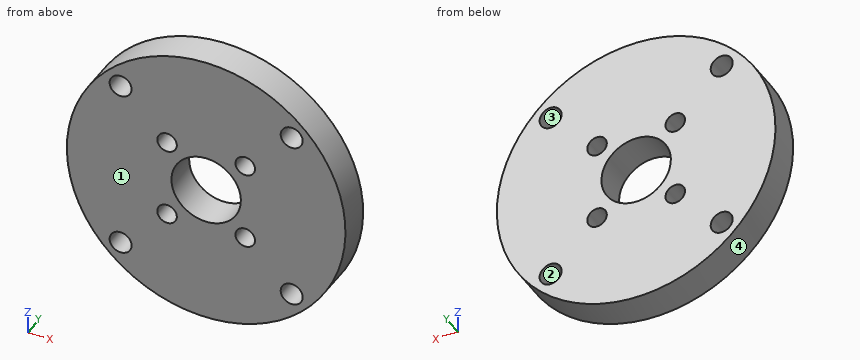
```python
from build123d import *

# Parameters (mm, degrees)
SKETCH1_R           = 28.5
BOSS_EXTRUDE1_DEPTH = 3.5
SKETCH2_R           = 2.25
SKETCH2_R_2         = 2
CUT_EXTRUDE1_DEPTH  = 41.908434338
SKETCH3_R           = 7.1
CUT_EXTRUDE2_DEPTH  = 41.908434338


with BuildPart() as part:
    # Sketch1 → Boss-Extrude1 (new, symmetric)
    with BuildSketch(Plane(origin=(0, 0, 0), x_dir=(1, 0, 0), z_dir=(0, 1, 0))):
        with Locations(Location((0, 0, 0), (0, 0, 270))):
            Circle(SKETCH1_R)
    extrude(amount=BOSS_EXTRUDE1_DEPTH, both=True)

    # Sketch2 → Cut-Extrude1 (cut, through all)
    with BuildSketch(Plane(origin=(0, 3.5, 0), x_dir=(1, 0, 0), z_dir=(0, 1, 0))):
        with Locations(Location((17.500892834, 17.500892834, 0), (0, 0, 270))):
            Circle(SKETCH2_R)
        with Locations(Location((17.500892834, -17.500892834, 0), (0, 0, 270))):
            Circle(SKETCH2_R)
        with Locations(Location((-17.500892834, -17.500892834, 0), (0, 0, 270))):
            Circle(SKETCH2_R)
        with Locations(Location((-17.500892834, 17.500892834, 0), (0, 0, 270))):
            Circle(SKETCH2_R)
        with Locations(Location((-8, -8, 0), (0, 0, 270))):
            Circle(SKETCH2_R_2)
        with Locations(Location((-8, 8, 0), (0, 0, 270))):
            Circle(SKETCH2_R_2)
        with Locations(Location((8, 8, 0), (0, 0, 270))):
            Circle(SKETCH2_R_2)
        with Locations(Location((8, -8, 0), (0, 0, 270))):
            Circle(SKETCH2_R_2)
    extrude(amount=-CUT_EXTRUDE1_DEPTH, mode=Mode.SUBTRACT)

    # Sketch3 → Cut-Extrude2 (cut, through all)
    with BuildSketch(Plane(origin=(0, 3.5, 0), x_dir=(1, 0, 0), z_dir=(0, 1, 0))):
        with Locations(Location((0, 0, 0), (0, 0, 270))):
            Circle(SKETCH3_R)
    extrude(amount=-CUT_EXTRUDE2_DEPTH, mode=Mode.SUBTRACT)


solid = part.part
```
Design review of the part built by this model. Coordinates are the model's own, in mm. Face numbers are marked on the shaded views. Coordinates: 2 decimals unless noted, no trailing zeros. Loops run counter-clockwise (first coordinate to the right, second up) from the corner with the lowest first, then second, coordinate; pieces in that order, holes last. Notation, with made-up numbers: (28.5, 47) - (45.5, 47) arc R23 cw to (45.5, 60) - close; hole circle Ø4 at (-6, 31). An arc over 180 degrees is marked (long way). Use CSV: the item, a comma, the result in double quotes. Start each with the question number.
1) Consider section A-A on x = 0. Write out the cut boundary in (y, z), then the cut area to 3 significant figures.
2) Consider section B-B on z = 0. Write out the cut boundary in (x, y).
3) Wall thickness on L1, parallel to X at y = 1.5, z = 0; L2, parallel to Z at x = -9, y = 2.5; L3, parallel to X at y = 2, z = 8: over which ranges is each line inside the solid? List them lowest first. Write a range as from..to.
4) The part is to be moulded in two halves that separate along Z. For the marked faces 1, 2, 3 and 4, say which applies: +Z half, -Z half, draft (parallel to the pull), parting line (faces both ways), or undercut.
5) For pin 1 Ø2.5 at (x, z) = (17.5, -17.5) entering from -Y; pin 2 Ø1 at (y, z) = (0.5, 13) entering from -X, all flat-tipped, find the tip position at first contact; note any pin that passes through.
6) Consider section D-D on x = 16.5. Write out the cut boundary in (y, z), then the cut area to 3 significant figures.
7) Consider section C-C on z = -8. Write out the cut boundary in (x, y).
Geometry says:
1,outline,"(-3.5, -28.5) - (3.5, -28.5) - (3.5, -7.1) - (-3.5, -7.1) - close; (-3.5, 7.1) - (3.5, 7.1) - (3.5, 28.5) - (-3.5, 28.5) - close"
1,area,"300 mm^2"
2,outline,"(-28.5, -3.5) - (-7.1, -3.5) - (-7.1, 3.5) - (-28.5, 3.5) - close; (7.1, -3.5) - (28.5, -3.5) - (28.5, 3.5) - (7.1, 3.5) - close"
3,L1,"-28.5..-7.1, 7.1..28.5"
3,L2,"-27.04..-9.73, -6.27..6.27, 9.73..27.04"
3,L3,"-27.35..-10, -6..6, 10..27.35"
4,face 1,"draft"
4,face 2,"undercut"
4,face 3,"undercut"
4,face 4,"parting line"
5,pin 1,"through"
5,pin 2,"x = -25.61"
6,outline,"(-3.5, -23.24) - (3.5, -23.24) - (3.5, -19.52) - (-3.5, -19.52) - close; (-3.5, -15.49) - (3.5, -15.49) - (3.5, 15.49) - (-3.5, 15.49) - close; (-3.5, 19.52) - (3.5, 19.52) - (3.5, 23.24) - (-3.5, 23.24) - close"
6,area,"269 mm^2"
7,outline,"(-27.35, -3.5) - (-10, -3.5) - (-10, 3.5) - (-27.35, 3.5) - close; (-6, -3.5) - (6, -3.5) - (6, 3.5) - (-6, 3.5) - close; (10, -3.5) - (27.35, -3.5) - (27.35, 3.5) - (10, 3.5) - close"
